Input: part model. Units: mm. Frame: model coordinates. A direction names the side the tool comes from. Coordinates: 2 decimals unless noted, no trailing zeros. Write each loop counter-clockwise with the first axis right and the second up, starting at its lowest first coordinate (ties: lowest second). Pieces come first, ordered by that corner, then holes. Notation, with made-up numbers: M 3,-25.75 L 50,-25.75 A33 ccw 50,6.25 Z; hole C 11.5,-10 d8. An arc over 180 degrees is marked long. Use one line per item in the form item = value.
from build123d import *

# Parameters (mm, degrees)
SKETCH010_W                                = 23.75
SKETCH010_H                                = 41.25
PAD003_DEPTH                               = 18
CHAMFER004013007011015006009007001028_SIZE = 3
SKETCH011_R                                = 1.9
POCKET007_DEPTH                            = 18.001
POCKET008_DEPTH                            = 13
FILLET_R                                   = 4
POCKET009_DEPTH                            = 18.001
FILLET001_R                                = 1
POCKET010_DEPTH                            = 23.751
FILLET002_R                                = 1
POCKET011_DEPTH                            = 18.001
FILLET003_R                                = 1
SKETCH016_R                                = 1.65
POCKET012_DEPTH                            = 41.251
SKETCH017_W                                = 6
SKETCH017_H                                = 3.2
SKETCH017_W_2                              = 3.75
PAD004_DEPTH                               = 1
CHAMFER004013007011015006009007001029_SIZE = 0.99
CHAMFER004013007011015006009007001030_SIZE = 0.6
CHAMFER004013007011015006009007001031_SIZE = 0.6


with BuildPart() as part:
    # Sketch010 → Pad003 (new body)
    with BuildSketch(Plane.XY):
        with Locations((11.875, -20.625)):
            Rectangle(SKETCH010_W, SKETCH010_H)
    extrude(amount=PAD003_DEPTH)

    # Chamfer004013007011015006009007001028
    chamfer004013007011015006009007001028_edges = [part.edges().sort_by_distance(p)[0] for p in [
        (11.875, 0, 0),
    ]]
    chamfer(chamfer004013007011015006009007001028_edges, length=CHAMFER004013007011015006009007001028_SIZE)

    # Sketch011 (on Face4 of Chamfer004013007011015006009007001028) → Pocket007 (cut, through all)
    with BuildSketch(Plane.XY.offset(18)):
        with Locations((18.75, -36.25)):
            Circle(SKETCH011_R)
    extrude(amount=-POCKET007_DEPTH, mode=Mode.SUBTRACT)

    # Sketch012 (on Face4 of Pocket007) → Pocket008 (cut)
    with BuildSketch(Plane.XY.offset(18)):
        with BuildLine():
            ThreePointArc((18.75, -30.25), (14.507359, -32.007359), (12.75, -36.25))
            Line((12.75, -41.25), (12.75, -36.25))
            Line((23.75, -41.25), (12.75, -41.25))
            Line((23.75, -30.25), (23.75, -41.25))
            Line((18.75, -30.25), (23.75, -30.25))
        make_face()
    extrude(amount=-POCKET008_DEPTH, mode=Mode.SUBTRACT)

    # Fillet
    fillet_edges = [part.edges().sort_by_distance(p)[0] for p in [
        (23.75, -41.25, 2.5),
    ]]
    fillet(fillet_edges, radius=FILLET_R)

    # Sketch013 (on Face8 of Fillet) → Pocket009 (cut, through all)
    with BuildSketch(Plane.XY.offset(18)):
        Polygon((0, -10), (0, -41.25), (8.75, -41.25), (8.75, -18.75), align=None)
    extrude(amount=-POCKET009_DEPTH, mode=Mode.SUBTRACT)

    # Fillet001
    fillet001_edges = [part.edges().sort_by_distance(p)[0] for p in [
        (8.75, -41.25, 9),
        (12.75, -41.25, 11.5),
        (23.75, -30.25, 11.5),
    ]]
    fillet(fillet001_edges, radius=FILLET001_R)

    # Sketch014 (on Face1 of Fillet001) → Pocket010 (cut, through all)
    with BuildSketch(Plane.YZ.offset(23.75)):
        Polygon((-42, 8), (-42, 19), (-4, 19), (-4, 13), (-9, 8), align=None)
    extrude(amount=-POCKET010_DEPTH, mode=Mode.SUBTRACT)

    # Fillet002
    fillet002_edges = [part.edges().sort_by_distance(p)[0] for p in [
        (0, -2, 18),
        (23.75, -2, 18),
    ]]
    fillet(fillet002_edges, radius=FILLET002_R)

    # Sketch015 (on Face14 of Fillet002) → Pocket011 (cut, through all)
    with BuildSketch(Plane.XY.offset(18)):
        Polygon((4, -4), (19.75, -4), (19.75, -26.25), (12, -26.25), (12, -17), (4, -9), align=None)
    extrude(amount=-POCKET011_DEPTH, mode=Mode.SUBTRACT)

    # Fillet003
    fillet003_edges = [part.edges().sort_by_distance(p)[0] for p in [
        (12, -26.25, 4),
        (19.75, -26.25, 4),
        (12, -17, 4),
    ]]
    fillet(fillet003_edges, radius=FILLET003_R)

    # Sketch016 (on Face26 of Fillet003) → Pocket012 (cut, through all)
    with BuildSketch(Plane(origin=(0, 0, 0), x_dir=(-1, 0, 0), z_dir=(0, 1, 0))):
        with Locations((-15.75, 10.5)):
            Circle(SKETCH016_R)
        with Locations((-8, 10.5)):
            Circle(SKETCH016_R)
    extrude(amount=-POCKET012_DEPTH, mode=Mode.SUBTRACT)

    # Sketch017 (on Face28 of Pocket012) → Pad004 (join)
    with BuildSketch(Plane(origin=(0, 0, 0), x_dir=(-1, 0, 0), z_dir=(0, 1, 0))):
        with Locations((-20.75, 10.5)):
            Rectangle(SKETCH017_W, SKETCH017_H)
        with Locations((-11.875, 10.5)):
            Rectangle(SKETCH017_W_2, SKETCH017_H)
        with Locations((-3, 10.5)):
            Rectangle(SKETCH017_W, SKETCH017_H)
    extrude(amount=PAD004_DEPTH)

    # Chamfer004013007011015006009007001029
    chamfer004013007011015006009007001029_edges = [part.edges().sort_by_distance(p)[0] for p in [
        (20.75, 1, 8.9),
        (11.875, 1, 8.9),
        (3, 1, 8.9),
    ]]
    chamfer(chamfer004013007011015006009007001029_edges, length=CHAMFER004013007011015006009007001029_SIZE)

    # Chamfer004013007011015006009007001030
    chamfer004013007011015006009007001030_edges = [part.edges().sort_by_distance(p)[0] for p in [
        (0, -6.5, 0),
        (4.375, -14.375, 0),
        (8.75, -29.5, 0),
        (9.042893, -40.957107, 0),
        (14.75, -41.25, 0),
        (22.578427, -40.078427, 0),
        (16.85, -36.25, 0),
        (23.75, -20.125, 0),
    ]]
    chamfer(chamfer004013007011015006009007001030_edges, length=CHAMFER004013007011015006009007001030_SIZE)

    # Chamfer004013007011015006009007001031
    chamfer004013007011015006009007001031_edges = [part.edges().sort_by_distance(p)[0] for p in [
        (11.875, -4, 0),
        (4, -6.5, 0),
        (7.853553, -12.853553, 0),
        (11.92388, -17.03153, 0),
        (12, -21.332107, 0),
        (12.292893, -25.957107, 0),
        (15.875, -26.25, 0),
        (19.457107, -25.957107, 0),
        (19.75, -14.625, 0),
    ]]
    chamfer(chamfer004013007011015006009007001031_edges, length=CHAMFER004013007011015006009007001031_SIZE)


solid = part.part
(1) Line query: probe 1 along Z at (x, y) = (15.75, -3); probe 2 along X at (y, z) = (-7, 4.5); probe 3 along Y at (x, z) = (18.75, 1.9). Output: solid intervals per line, ascending.
Computed:
probe_1 = 0 to 8.85, 12.15 to 18
probe_2 = 0 to 4, 19.75 to 23.75
probe_3 = -41.25 to -38.15, -34.35 to -26.25, -4 to -1.1
(2) Set-up query: faces 1 (the conical face through (12.14, -26.13, 0.37)), 2 (the flat face through (11, -24, 8)), 3 (the cylindrical face through (19.465, -25.949, 4.248)), 4 (the flat face through (10, 0.5, 10.8)), 5 (the flat face through (21, -30.25, 7)). Return all of +Z, -Z, +X, -X, +Y, -Y with unobstructed straight access to the full face (end or side cutting, diameter ignored); none if empty.
Computed:
face_1 = -Z
face_2 = +Z, +X, -X, -Y
face_3 = +Z, -Z
face_4 = +Z, -Z, +Y
face_5 = +Z, +X, -Y
(3) First-contact query: pin 1 Ø3 at (x, z) = (17, 3.5) entering from +Y; pin 2 Ø1.5 at (y, z) = (-28, 4) entering from -X; pin 3 Ø4 at (x, y) = (18, -23.5) entering from -Z; pin 4 Ø6 at (x, y) = (15, -12.5) entering from +Z. Flat tips, straight axial feed; report the tip coordinate or a pass-through.
Computed:
pin_1 = 0
pin_2 = 8.75
pin_3 = 0.35
pin_4 = through
(4) Section query D-D on z = 11. Return the cut outline in (x, y), plus the area to 3 significant figures.
Computed:
outline = M 0,-6 L 4,-6 L 4,-4 L 6.43,-4 L 6.43,0 L 6,0 L 6,1 L 0,1 Z; M 9.57,-4 L 14.18,-4 L 14.18,0 L 13.75,0 L 13.75,1 L 10,1 L 10,0 L 9.57,0 Z; M 17.32,-4 L 19.75,-4 L 19.75,-6 L 23.75,-6 L 23.75,1 L 17.75,1 L 17.75,0 L 17.32,0 Z
area = 102 mm^2
(5) Section query B-B on y = -22. Return the cut outline in (x, z), plus the area to 3 significant figures.
Computed:
outline = M 8.75,0.6 L 9.35,0 L 11.4,0 L 12,0.6 L 12,8 L 8.75,8 Z; M 19.75,0.6 L 20.35,0 L 23.15,0 L 23.75,0.6 L 23.75,8 L 19.75,8 Z
area = 57.3 mm^2
(6) Section query C-C on x = 15.75. Return the cut outline in (y, z).
Computed:
outline = M -41.25,0.6 L -40.65,0 L -26.85,0 L -26.25,0.6 L -26.25,8 L -31.05,8 L -31.05,5 L -41.25,5 Z; M -4,0.6 L -3.4,0 L -3,0 L 0,3 L 0,8.85 L -4,8.85 Z; M -4,12.15 L 0,12.15 L 0,18 L -4,18 Z
(7) Section query A-A on z = 4. Return the cut outline in (x, y), plus the area to 3 significant figures.
Computed:
outline = M 0,-10 L 8.75,-18.75 L 8.75,-40.25 A1 ccw 9.75,-41.25 L 19.75,-41.25 A4 ccw 23.75,-37.25 L 23.75,0 L 0,0 Z; hole M 4,-9 L 11.71,-16.71 A1 cw 12,-17.41 L 12,-25.25 A1 ccw 13,-26.25 L 18.75,-26.25 A1 ccw 19.75,-25.25 L 19.75,-4 L 4,-4 Z; hole C 18.75,-36.25 d3.8
area = 486 mm^2
(8) Pull-direction query (X, two-part tool) for faces 6 (the flat face through (8, -13, 4)), 7 (the flat face through (20.79, 0.51, 9.4)), 8 (the cylindrical face through (23.465, -1.972, 17.699)), 9 (the flat face through (4, -14, 4)); classes: pulls with the +X half, pulls with the -X half, needs draft (parallel to the pull), parting line crosses it, or undercut.
Computed:
face_6 = undercut
face_7 = needs draft
face_8 = pulls with the +X half
face_9 = pulls with the -X half
